The model under review builds one solid part; all positions refer to its coordinate system, in mm. Round coordinates to 2 decimals unless told otherwise and drop trailing zeros. Write each loop counter-clockwise with the first axis right and the second up, starting at its lowest first coordinate (ties: lowest second). Pieces come first, ordered by that corner, then holes. Notation, with made-up numbers: (63.5, -12) -> (101.5, -12) arc R18 ccw to (101.5, 9) -> close; hole circle Ø10 at (69, 38.25). An arc over 180 degrees is marked (long way). Return JSON: item names as keys, results as strings. Group by question number.
1. Take a section at A-A, the plane y = 0.5. Write out the cut boundary in (x, z).
2. For line 1 along Z through (x, y) = (9.75, 1.2); line 2 along X through (y, z) = (0.15, 3.75), list the stretches that pass through material, from the lowest coordinate up. Write a range as from..to.
3. Clearance check with flat-ended pins moving along their axes: P1, Ø0.7, axis at x = -6.5, y = 1, coming from the -Z side; P2, Ø0.7, axis at y = 0.5, z = -8, coming from the -X side; P3, Ø0.7, axis at y = 0.5, z = 4, coming from the +X side. State where each tip first meets the part, or that it passes through.
4. Take a section at B-B, the plane x = -5.5. Write out the cut boundary in (y, z).
Autodesk Inventor part; units mm, degrees
ref_plane "YZ Plane" through (0, 0, 0) normal (1, 0, 0) x (0, 1, 0)
ref_plane "XZ Plane" through (0, 0, 0) normal (0, 1, 0) x (-1, 0, 0)
ref_plane "XY Plane" through (0, 0, 0) normal (0, 0, 1) x (1, 0, 0)
sketch "Esquisse1" plane through (0, 0, 0) normal (0, 1, 0) x (-1, 0, 0)
  line L0 (4.9536, 5.2597) -> (4.9536, 3.2597)
  line L1 (4.9536, 3.2597) -> (6.9536, 3.2597)
  line L2 (-9.0464, 5.2597) -> (-9.0464, 3.2597)
  line L3 (-9.0464, 3.2597) -> (-11.0464, 3.2597)
  line L4 (-9.0464, -8.7403) -> (-9.0464, -6.7403)
  line L5 (-9.0464, -6.7403) -> (-11.0464, -6.7403)
  line L6 (4.9536, -8.7403) -> (4.9536, -6.7403)
  line L7 (4.9536, -6.7403) -> (6.9536, -6.7403)
  line L8 (4.9536, 5.2597) -> (-9.0464, 5.2597)
  line L9 (-11.0464, 3.2597) -> (-11.0464, -6.7403)
  line L10 (-9.0464, -8.7403) -> (4.9536, -8.7403)
  line L11 (6.9536, -6.7403) -> (6.9536, 3.2597)
  point P0 (0, 0)
  dimension "d2" = 2
  dimension "d3" = 2
  dimension "d4" = 2
  dimension "d5" = 2
  dimension "d6" = 2
  dimension "d7" = 2
  dimension "d8" = 2
  dimension "d9" = 2
  dimension "d16" = 10
  dimension "d17" = 18
extrude "Extrusion1" add sketch "Esquisse1" along normal blind 1.4
properties part number "pcb"
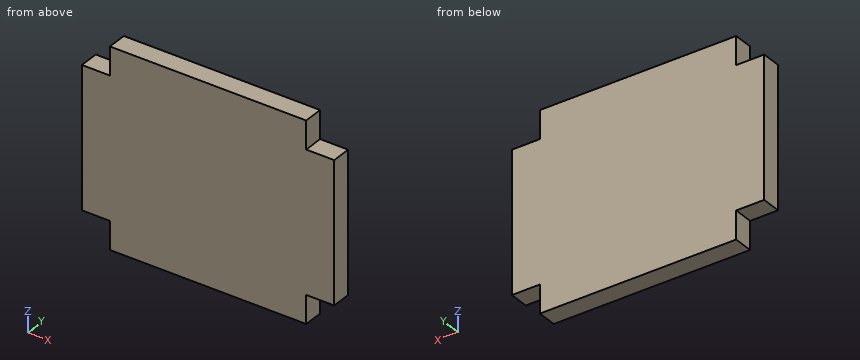
Output:
{
 "1": {"outline": "(-6.95, -6.74) -> (-4.95, -6.74) -> (-4.95, -8.74) -> (9.05, -8.74) -> (9.05, -6.74) -> (11.05, -6.74) -> (11.05, 3.26) -> (9.05, 3.26) -> (9.05, 5.26) -> (-4.95, 5.26) -> (-4.95, 3.26) -> (-6.95, 3.26) -> close"},
 "2": {"line 1": "z = -6.74..3.26", "line 2": "x = -4.95..9.05"},
 "3": {"P1": "stops at z = -6.74", "P2": "stops at x = -4.95", "P3": "stops at x = 9.05"},
 "4": {"outline": "(0, -6.74) -> (1.4, -6.74) -> (1.4, 3.26) -> (0, 3.26) -> close"}
}
